from build123d import *

# Parameters (mm, degrees)
SKETCH1_R           = 26.797
BOSS_EXTRUDE1_DEPTH = 3.5
SKETCH2_R           = 25.9969
BOSS_EXTRUDE2_DEPTH = 24
SKETCH3_R           = 25.9969
BOSS_EXTRUDE3_DEPTH = 24
SKETCH4_R           = 7.625
CUT_EXTRUDE1_DEPTH  = 24
SKETCH5_R           = 7.625
SKETCH5_R_2         = 4.490128061
CUT_EXTRUDE2_DEPTH  = 24
SKETCH6_R           = 5.25
SKETCH6_R_2         = 5
CUT_EXTRUDE4_DEPTH  = 52.5
CUT_EXTRUDE5_START  = -26.797
SKETCH7_W           = 16.5
SKETCH7_H           = 5.75
CUT_EXTRUDE5_DEPTH  = 25.9969
CUT_EXTRUDE6_DEPTH  = 5.75
SKETCH13_W          = 16.5
SKETCH13_H          = 9.75
CUT_EXTRUDE10_DEPTH = 12.797
CUT_EXTRUDE11_DEPTH = 9.75
SKETCH9_W           = 23
SKETCH9_H           = 4.25
CUT_EXTRUDE7_DEPTH  = 12.797
CUT_EXTRUDE8_DEPTH  = 4.25
CUT_EXTRUDE9_START  = -12.797
SKETCH12_W          = 10.5
SKETCH12_H          = 2
CUT_EXTRUDE9_DEPTH  = 11.9969


with BuildPart() as part:
    # Sketch1 → Boss-Extrude1 (new body)
    with BuildSketch(Plane(origin=(0, 0, 0), x_dir=(1, 0, 0), z_dir=(0, 1, 0))):
        Circle(SKETCH1_R)
    extrude(amount=BOSS_EXTRUDE1_DEPTH)

    # Sketch2 → Boss-Extrude2 (add)
    with BuildSketch(Plane(origin=(0, 3.5, 0), x_dir=(1, 0, 0), z_dir=(0, 1, 0))):
        Circle(SKETCH2_R)
    extrude(amount=BOSS_EXTRUDE2_DEPTH)

    # Sketch3 → Boss-Extrude3 (add)
    with BuildSketch(Plane.XZ):
        Circle(SKETCH3_R)
    extrude(amount=BOSS_EXTRUDE3_DEPTH)

    # Sketch4 → Cut-Extrude1 (cut)
    with BuildSketch(Plane.XZ.offset(24)):
        with Locations((-13.255925111, -8.959935794)):
            Circle(SKETCH4_R)
        with Locations((13.255925111, -8.959935794)):
            Circle(SKETCH4_R)
    extrude(amount=-CUT_EXTRUDE1_DEPTH, mode=Mode.SUBTRACT)

    # Sketch5 → Cut-Extrude2 (cut)
    with BuildSketch(Plane(origin=(0, 27.5, -30.35), x_dir=(-1, 0, 0), z_dir=(0, -1, 0))):
        with Locations((-13.255925111, -21.390064206)):
            Circle(SKETCH5_R)
        with Locations((13.255925111, -21.390064206)):
            Circle(SKETCH5_R)
        with Locations((0, -30.35)):
            Circle(SKETCH5_R_2)
    extrude(amount=CUT_EXTRUDE2_DEPTH, mode=Mode.SUBTRACT)

    # Sketch6 → Cut-Extrude4 (cut, through all)
    with BuildSketch(Plane(origin=(0, -24, -24), x_dir=(-1, 0, 0), z_dir=(0, 1, 0))):
        with Locations((0, 38)):
            Circle(SKETCH6_R)
        with Locations((-13.255925111, 15.040064206)):
            Circle(SKETCH6_R_2)
        with Locations((13.255925111, 15.040064206)):
            Circle(SKETCH6_R_2)
    extrude(amount=CUT_EXTRUDE4_DEPTH, mode=Mode.SUBTRACT)

    # Sketch7 → Cut-Extrude5 (cut)
    with BuildSketch(Plane.XY.offset(26.797).offset(CUT_EXTRUDE5_START)):
        with Locations((0, 6.375)):
            Rectangle(SKETCH7_W, SKETCH7_H)
    extrude(amount=CUT_EXTRUDE5_DEPTH, mode=Mode.SUBTRACT)

    # Sketch8 → Cut-Extrude6 (cut)
    with BuildSketch(Plane(origin=(0, 3.5, 0), x_dir=(1, 0, 0), z_dir=(0, 1, 0))):
        with BuildLine():
            Line((-8.25, 0), (8.25, 0))
            ThreePointArc((8.25, 0), (0, 8.25), (-8.25, 0))
        make_face()
    extrude(amount=CUT_EXTRUDE6_DEPTH, mode=Mode.SUBTRACT)

    # Sketch13 → Cut-Extrude10 (cut)
    with BuildSketch(Plane.XY.offset(26.797)):
        with Locations((0, -1.375)):
            Rectangle(SKETCH13_W, SKETCH13_H)
    extrude(amount=-CUT_EXTRUDE10_DEPTH, mode=Mode.SUBTRACT)

    # Sketch14 → Cut-Extrude11 (cut)
    with BuildSketch(Plane(origin=(0, -6.25, 0), x_dir=(1, 0, 0), z_dir=(0, 1, 0))):
        with BuildLine():
            Line((-8.25, -14), (8.25, -14))
            ThreePointArc((8.25, -14), (0, -5.75), (-8.25, -14))
        make_face()
    extrude(amount=CUT_EXTRUDE11_DEPTH, mode=Mode.SUBTRACT)

    # Sketch9 → Cut-Extrude7 (cut)
    with BuildSketch(Plane.XY.offset(26.797)):
        with Locations((0, -8.375)):
            Rectangle(SKETCH9_W, SKETCH9_H)
    extrude(amount=-CUT_EXTRUDE7_DEPTH, mode=Mode.SUBTRACT)

    # Sketch11 → Cut-Extrude8 (cut)
    with BuildSketch(Plane(origin=(0, -10.5, 0), x_dir=(1, 0, 0), z_dir=(0, 1, 0))):
        with BuildLine():
            Line((-11.5, -14), (11.5, -14))
            ThreePointArc((11.5, -14), (0, -2.5), (-11.5, -14))
        make_face()
    extrude(amount=CUT_EXTRUDE8_DEPTH, mode=Mode.SUBTRACT)

    # Sketch12 → Cut-Extrude9 (cut)
    with BuildSketch(Plane.XY.offset(26.797).offset(CUT_EXTRUDE9_START)):
        with Locations((0, -11.5)):
            Rectangle(SKETCH12_W, SKETCH12_H)
    extrude(amount=CUT_EXTRUDE9_DEPTH, mode=Mode.SUBTRACT)


solid = part.part
Work out the finished part from the listing and answer in its coordinate system (mm). A direction names the side the tool comes from. Give positions to 0.01 mm unless a question says otherwise; leave off trailing zeros. Loops run counter-clockwise (first coordinate to the right, second up) from the corner with the lowest first, then second, coordinate; pieces in that order, holes last. Notation, with made-up numbers: (21.25, 69) - (41.25, 69) arc R27 ccw to (41.25, 106) - close; hole circle Ø7 at (42.5, 25). An arc over 180 degrees is marked (long way). Answer in a Markdown table with one row per item.
(1) Flat-ended cylindrical pins translate along their axes: pin 1 Ø3.5 at (y, z) = (-9, 19) entering from +X; pin 2 Ø1.3 at (y, z) = (-8, 20) entering from -X; pin 3 Ø8 at (x, y) = (9.5, -18) entering from -Z. Find the tip coordinate at first contact, or state that the pin passes through.
Results list:
| item | result |
|---|---|
| pin 1 | stops at x = 19.45 |
| pin 2 | stops at x = -17.36 |
| pin 3 | stops at z = -25.41 |
(2) Section A-A (x = 0) is taken. Give the vertices of the cut face in (y, z).
Results list:
| item | result |
|---|---|
| outline | (-24, -26) - (0, -26) - (0, -26.8) - (3.5, -26.8) - (3.5, -26) - (27.5, -26) - (27.5, -4.49) - (9.25, -4.49) - (9.25, -8.25) - (3.5, -8.25) - (3.5, 5.75) - (-6.25, 5.75) - (-6.25, 2.5) - (-10.5, 2.5) - (-10.5, 8.75) - (-24, 8.75) - close; (-24, 19.25) - (-12.5, 19.25) - (-12.5, 26) - (-24, 26) - close; (9.25, 4.49) - (27.5, 4.49) - (27.5, 8.75) - (9.25, 8.75) - close; (9.25, 19.25) - (27.5, 19.25) - (27.5, 26) - (9.25, 26) - close |
(3) Consider L1, parallel to Z at x = 0, y = 15.25; L2, parallel to X at y = 13.5, z = 0; L3, parallel to Y at x = -7, z = 5.5. Determine where each line is inside the solid, lowest interval first. Write a range as [from, to].
Results list:
| item | result |
|---|---|
| L1 | z = [-26, -4.49], [4.49, 8.75], [19.25, 26] |
| L2 | x = [-26, -4.49], [4.49, 26] |
| L3 | y = [-24, -10.5], [-6.25, 3.5], [9.25, 27.5] |
(4) For a pull along X with two mould halves and no side action, classify faces 1 (the face through (-14, 0, -22.1)), 2 (the face through (-5.636, -11.832, -25.379)), 3 (the face through (20.53, -12.17, -6.67)) as pulls with the +X half, pulls with the -X half, needs draft (parallel to the pull), parting line crosses it, or undercut.
Results list:
| item | result |
|---|---|
| face 1 | needs draft |
| face 2 | parting line crosses it |
| face 3 | undercut |
(5) A tool of negligible diameter and unlimited length cuts with its end or side. For faces 4 (the face through (3.563, 18.503, 2.732)), 5 (the face through (0, 3.5, 0)), 6 (the face through (-6.212, -12.168, -11.88)), from which of +Z, -Z, +X, -X, +Y, -Y can it reach the whole face along a straight path? Write none if from no direction.
Results list:
| item | result |
|---|---|
| face 4 | +Y |
| face 5 | +Z |
| face 6 | -Y |
(6) Section D-D (y = 6.5) is taken. Give the vertices of the cut face in (x, z) (3 decimals), and give its area (3 significant figures).
Results list:
| item | result |
|---|---|
| outline | (-8.25, 0) - (-8.25, 24.653) arc R25.997 ccw (long way) to (8.25, 24.653) - (8.25, 0) arc R8.25 cw to start; hole circle Ø15.25 at (-13.256, -8.96); hole circle Ø15.25 at (13.256, -8.96) |
| area | 1,230 mm² |
(7) Section C-C (x = 13) is taken. Give the vertices of the cut face in (y, z), and give its area (3 significant figures).
Results list:
| item | result |
|---|---|
| outline | (-24, -22.51) - (0, -22.51) - (0, -23.43) - (3.5, -23.43) - (3.5, -22.51) - (27.5, -22.51) - (27.5, -16.58) - (3.5, -16.58) - (3.5, -13.95) - (0, -13.95) - (0, -16.58) - (-24, -16.58) - close; (-24, -1.34) - (0, -1.34) - (0, -3.97) - (3.5, -3.97) - (3.5, -1.34) - (27.5, -1.34) - (27.5, 22.51) - (3.5, 22.51) - (3.5, 23.43) - (0, 23.43) - (0, 22.51) - (-24, 22.51) - close |
| area | 1,560 mm² |
